Geometry: see drawing. Coordinates: mm, zero at the bounding-box minimum. Round coordinates to 2 decimals unless told otherwise and drop trailing zeros. Loops run counter-clockwise (first coordinate to the right, second up) from the corner with the lowest first, then second, coordinate; pieces in that order, holes last. Notation, with made-up numbers: M 22,24 L 70,24 A19 ccw 70,37 Z; hole C 53,-31 d2. An arc over 180 degrees is marked long. Answer as a JSON object with one key per item and string values.
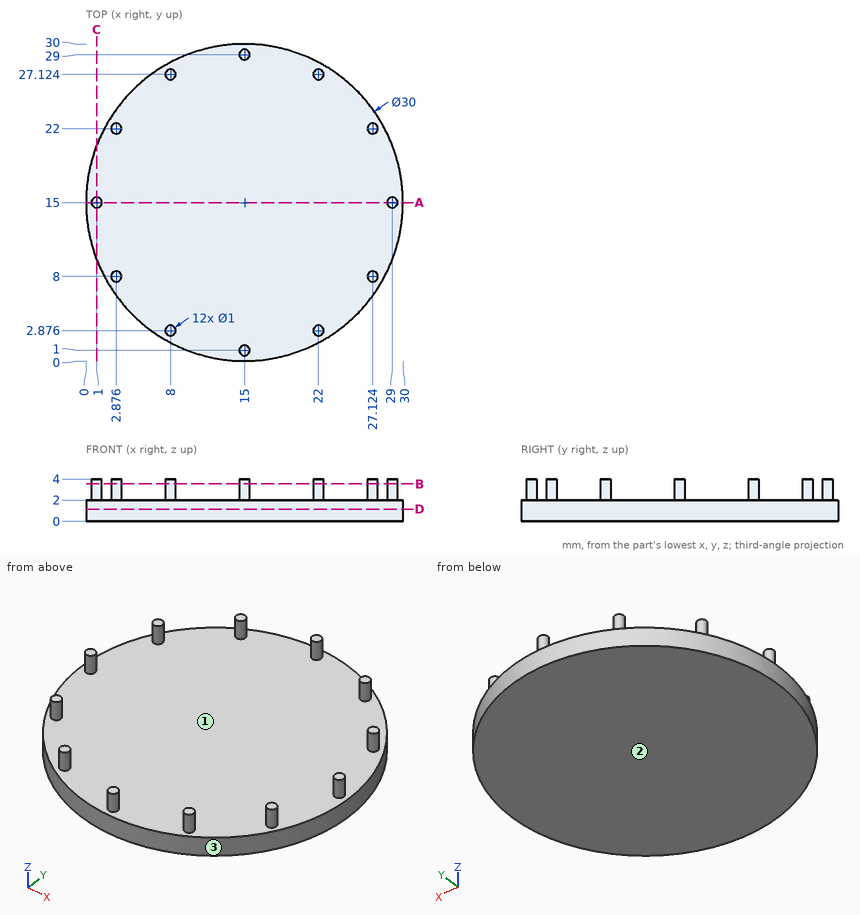
1) Section query C-C (x = 1). Return the cut outline in (y, z) (1 decimal).
Results:
{"outline": "M 9.6,0 L 20.4,0 L 20.4,2 L 15.5,2 L 15.5,4 L 14.5,4 L 14.5,2 L 9.6,2 Z"}
2) Section query B-B (z = 3.55). Count the separate pieces of the cut face and the enclosed holes in it.
Results:
{"separate pieces": "12", "enclosed holes": "0"}
3) Pin query (flat end, axial travel): P1, Ø1, axis at x = 16.5, y = 21, coming from the +Z side; P2, Ø2, axis at y = 20, z = 0.5, coming from the +X side. Return the tip coordinate at first contact, or that it passes through.
Results:
{"P1": "z = 2", "P2": "x = 29.46"}
4) Section query A-A (y = 15). Return the cut outline in (x, z).
Results:
{"outline": "M 0,0 L 30,0 L 30,2 L 29.5,2 L 29.5,4 L 28.5,4 L 28.5,2 L 1.5,2 L 1.5,4 L 0.5,4 L 0.5,2 L 0,2 Z"}
5) Pull-direction query (Y, two-part tool) for the marked faces 1, 2 and 3; classes: +Y half, -Y half, draft (parallel to the pull), parting line (faces both ways), or undercut.
Results:
{"face 1": "undercut", "face 2": "draft", "face 3": "parting line"}
6) Section query D-D (z = 1.15). Return the cut outline in (x, y).
Results:
{"outline": "C 15,15 d30"}
7) Ray query, line 1 (Z direction, x = 14.75, y = 27); line 2 (X direction, y = 2.75, z = 2.6) (1 decimal); line 3 (Y direction, x = 16.25, z = 1). Return the intervals inside material, ascending.
Results:
{"line 1": "0 to 2", "line 2": "7.5 to 8.5, 21.5 to 22.5", "line 3": "0.05 to 29.95"}
